Part model, mm, in its own coordinate system. Face numbers are marked on the shaded views. A direction names the side the tool comes from. Round coordinates to 2 decimals unless told otherwise and drop trailing zeros. Write each loop counter-clockwise with the first axis right and the second up, starting at its lowest first coordinate (ties: lowest second). Pieces come first, ordered by that corner, then holes. Notation, with made-up numbers: (89.25, 41.25) -> (122.25, 41.25) arc R15 cw to (122.25, 62.25) -> close; hole circle Ø4 at (89, 9). An arc over 180 degrees is marked (long way). Use CSV: the item, a comma, the result in double quotes. Start each with the question number.
(1) Saw through at C-C (y = 77). Give the cut face in (x, z) (3 decimals).
(2) Saw through at B-B (x = 134.5). Give the cut face in (y, z) (1 decimal), plus the area to 3 significant figures.
(3) Saw through at D-D (z = -22). Give the cut face in (x, y), plus the area to 3 significant figures.
(4) Drop flat-ended pins along their axis: pin 1 (20.5 mm diameter, centred on x = 88.77, y = 52.26, fed in from +Z); pin 2 (12 mm diameter, centred on x = 44.5, y = 82.5, fed in from +Z). Give the stop position or say it passes through.
(5) Probe line 1 (Y direction, x = 136, z = -10); line 2 (X direction, y = 88.5, z = -9.5); line 3 (X direction, y = 53, z = -40). List the from-to ranges inside material, lowest first. Write a range as [from, to].
(6) Which spindle directions (+Z, -Z, +X, -X, +Y, -Y) get a long thin tool onto all of the face, cutting with end or side? Do the marked faces 5 and 6. Say none if no direction does.
(7) Two-plate mould, pull along X, no slides. Class the marked faces 1, 2, 3 and 4: released by +X, released by -X, zero draft, split by the parting line, or undercut.
(8) Saw through at A-A (z = -10). Give the cut face in (x, y), plus the area to 3 significant figures.
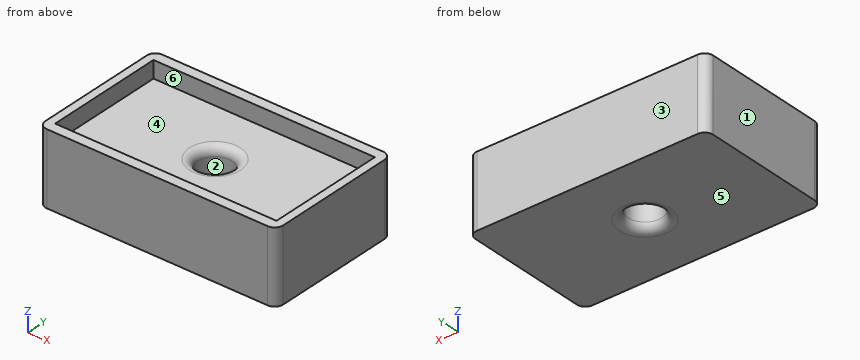
```python
from build123d import *

# Parameters (mm, degrees)
F0_W     = 177.546
F0_H     = 104.521
F0_W_2   = 165.354
F0_H_2   = 89.154
F0_R     = 12.7
F1_DEPTH = 53.975
F2_DEPTH = 12.7
F3_R     = 6.35


with BuildPart() as f1:
    # F0 (on Top) → F1 (new body)
    with BuildSketch(Plane.XY):
        with Locations((88.773, 52.2605)):
            Rectangle(F0_W, F0_H)
        with Locations((88.773, 52.2605)):
            Rectangle(F0_W_2, F0_H_2, mode=Mode.SUBTRACT)
        with Locations((88.773, 52.2605)):
            Rectangle(F0_W_2, F0_H_2)
        with Locations((88.773, 52.2605)):
            Circle(F0_R, mode=Mode.SUBTRACT)
    extrude(amount=-F1_DEPTH)

    # F0 (on Top) → F2 (cut)
    with BuildSketch(Plane.XY):
        with Locations((88.773, 52.2605)):
            Rectangle(F0_W_2, F0_H_2)
        with Locations((88.773, 52.2605)):
            Circle(F0_R, mode=Mode.SUBTRACT)
    extrude(amount=-F2_DEPTH, mode=Mode.SUBTRACT)

    # F3
    f3_edges = [f1.edges().sort_by_distance(p)[0] for p in [
        (0, 0, -26.9875),
        (177.546, 104.521, -26.9875),
        (177.546, 0, -26.9875),
        (0, 104.521, -26.9875),
        (76.073, 52.2605, -12.7),
        (76.073, 52.2605, -53.975),
    ]]
    fillet(f3_edges, radius=F3_R)


solid = f1.part
```
Answers:
1,outline,"(0, -53.975) -> (177.546, -53.975) -> (177.546, 0) -> (171.45, 0) -> (171.45, -12.7) -> (6.096, -12.7) -> (6.096, 0) -> (0, 0) -> close"
2,outline,"(0, -54) -> (104.5, -54) -> (104.5, 0) -> (96.8, 0) -> (96.8, -12.7) -> (7.7, -12.7) -> (7.7, 0) -> (0, 0) -> close"
2,area,"4,510 mm²"
3,outline,"(0, 6.35) arc R6.35 ccw to (6.35, 0) -> (171.2, 0) arc R6.35 ccw to (177.55, 6.35) -> (177.55, 98.17) arc R6.35 ccw to (171.2, 104.52) -> (6.35, 104.52) arc R6.35 ccw to (0, 98.17) -> close; hole circle Ø25.4 at (88.77, 52.26)"
3,area,"18,000 mm²"
4,pin 1,"passes through"
4,pin 2,"stops at z = -12.7"
5,line 1,"y = [0, 7.68], [96.84, 104.52]"
5,line 2,"x = [0, 6.1], [171.45, 177.55]"
5,line 3,"x = [0, 76.09], [101.45, 177.55]"
6,face 5,"-Z, +X, -X, +Y, -Y"
6,face 6,"+Z"
7,face 1,"released by -X"
7,face 2,"undercut"
7,face 3,"zero draft"
7,face 4,"undercut"
8,outline,"(0, 6.35) arc R6.35 ccw to (6.35, 0) -> (171.2, 0) arc R6.35 ccw to (177.55, 6.35) -> (177.55, 98.17) arc R6.35 ccw to (171.2, 104.52) -> (6.35, 104.52) arc R6.35 ccw to (0, 98.17) -> close; hole (6.1, 7.68) -> (171.45, 7.68) -> (171.45, 96.84) -> (6.1, 96.84) -> close"
8,area,"3,780 mm²"
